For this review, take the finished solid that the model builds, in its own axes (mm). A direction names the side the tool comes from. Give positions to 0.01 mm unless a question says otherwise; leave off trailing zeros. Write each loop counter-clockwise with the first axis right and the second up, starting at its lowest first coordinate (ties: lowest second). Pieces come first, ordered by that corner, then holes.
Q1. We need section C-C (z = 0.4). Write out the cut boundary in (x, y), then the cut area to 3 significant figures.
Q2. Machinability: for faces 5 (the flat face through (-1, 2, 0)), 6 (the flat face through (2, -2, 2.9)), which of the approach directions +Z, -Z, +X, -X, +Y, -Y give a long, thin tool a straight path to every point of the face, cutting with its end or side? Answer none if there is none.
Q3. We need section A-A (y = 0). Write out the cut boundary in (x, z), then the cut area to 3 significant figures.
Q4. Insertion check: P1, Ø1.5, axis at x = -2, z = 0.5, coming from the -Y side. The pin has a flat end and moves straight along its axis. Give the tip position at first contact, or say it passes through.
Q5. Mouldability with a two-part tool opening along Y and no side actions: class faces 1 (the flat face through (-1, 2, 3)), 2 (the cylindrical face through (-0.867, 3.905, 1.783)), 3 (the cylindrical face through (0, 2, 1)), 4 (the flat face through (-2, -2, 0.1)) as released by +Y, released by -Y, zero draft, split by the parting line, or undercut.
Q6. For line 1 (Y direction, x = 0, z = 2.95); line 2 (Y direction, x = 0, z = 0.85); line 3 (X direction, y = -1.5, z = 2.6), list the stretches that pass through material, from the lowest coordinate up.
Q7. We need section D-D (x = 2.25). Write out the cut boundary in (y, z).
Autodesk Inventor part; units mm, degrees
ref_plane "YZ Plane" through (0, 0, 0) normal (1, 0, 0) x (0, 1, 0)
ref_plane "XZ Plane" through (0, 0, 0) normal (0, 1, 0) x (-1, 0, 0)
ref_plane "XY Plane" through (0, 0, 0) normal (0, 0, 1) x (1, 0, 0)
sketch "スケッチ1" plane through (0, 0, 0) normal (0, 0, 1) x (1, 0, 0)
  circle A0 centre (0, 0) radius 2
  circle A1 centre (0, 0) radius 4
  circle A2 centre (0, 0) radius 4.6
  dimension "d0" = 4
  dimension "d1" = 8
  dimension "d2" = 0.6
extrude "押し出し1" add sketch "スケッチ1" along normal blind 3 contours A1
extrude "押し出し2" add sketch "スケッチ1" along normal blind 0.6 contours A2
sketch "スケッチ2" plane through (0, 0, 0) normal (0, 0, -1) x (-1, 0, 0)
  circle A0 centre (0, 0) radius 2.5
  circle A1 centre (0, 0) radius 3.5
  dimension "d7" = 5
  dimension "d8" = 7
extrude "押し出し3" cut sketch "スケッチ2" against normal blind 0.1
sketch "スケッチ3" plane through (0, 0, 3) normal (0, 0, 1) x (1, 0, 0)
  circle A0 centre (0, 0) radius 2.5
  circle A1 centre (0, 0) radius 3.5
  dimension "d11" = 5
  dimension "d12" = 7
extrude "押し出し4" cut sketch "スケッチ3" against normal blind 0.1
properties part number "ベアリングd4D8B3F" material "鋼、炭素鋼"
Computed:
1. outline: circle Ø9.2 at (0, 0); hole circle Ø4 at (0, 0)
1. area: 53.9 mm2
2. face 5: -Z, +X, -X, +Y, -Y
2. face 6: +Z
3. outline: (-4.6, 0) - (-3.5, 0) - (-3.5, 0.1) - (-2.5, 0.1) - (-2.5, 0) - (-2, 0) - (-2, 3) - (-2.5, 3) - (-2.5, 2.9) - (-3.5, 2.9) - (-3.5, 3) - (-4, 3) - (-4, 0.6) - (-4.6, 0.6) - close; (2, 0) - (2.5, 0) - (2.5, 0.1) - (3.5, 0.1) - (3.5, 0) - (4.6, 0) - (4.6, 0.6) - (4, 0.6) - (4, 3) - (3.5, 3) - (3.5, 2.9) - (2.5, 2.9) - (2.5, 3) - (2, 3) - close
3. area: 12.3 mm2
4. P1: stops at y = -4.43
5. face 1: zero draft
5. face 2: split by the parting line
5. face 3: undercut
5. face 4: undercut
6. line 1: y = -4 to -3.5, -2.5 to -2, 2 to 2.5, 3.5 to 4
6. line 2: y = -4 to -2, 2 to 4
6. line 3: x = -3.71 to -1.32, 1.32 to 3.71
7. outline: (-4.01, 0) - (-2.68, 0) - (-2.68, 0.1) - (-1.09, 0.1) - (-1.09, 0) - (1.09, 0) - (1.09, 0.1) - (2.68, 0.1) - (2.68, 0) - (4.01, 0) - (4.01, 0.6) - (3.31, 0.6) - (3.31, 3) - (2.68, 3) - (2.68, 2.9) - (1.09, 2.9) - (1.09, 3) - (-1.09, 3) - (-1.09, 2.9) - (-2.68, 2.9) - (-2.68, 3) - (-3.31, 3) - (-3.31, 0.6) - (-4.01, 0.6) - close
